Input: part model. Units: mm. Frame: model coordinates. Face numbers are marked on the shaded views. A direction names the side the tool comes from. Coordinates: 2 decimals unless noted, no trailing zeros. Write each loop counter-clockwise with the first axis right and the second up, starting at its lowest first coordinate (ties: lowest second). Pieces come first, ordered by that corner, then holes. Notation, with made-up numbers: M -2.75,24.5 L 14.25,24.5 A9 ccw 14.25,34.5 Z; hole C 26.5,47 d7. An arc over 180 degrees is marked long. Write each question's results on one line, items separated by ' | '. Start each with the question number.
1. Section query A-A, the plane x = 33. Output: boundary loops of the cut face in (y, z), and give its area (3 significant figures).
2. Ray query, probe 1 along Z at (x, y) = (15, -3); probe 2 along X at (y, z) = (-2.25, 6.25); probe 3 along Z at (x, y) = (30, 0). Return the intervals inside material, ascending.
3. Set-up query: the marked faces 1 and 2. Return all of +Z, -Z, +X, -X, +Y, -Y with unobstructed straight access to the full face (end or side cutting, diameter ignored); none if empty.
4. First-contact query: pin 1 (2 mm diameter, centred on x = 41, y = -2, fed in from -Z); pin 2 (4 mm diameter, centred on y = 3, z = -6, fed in from +X); pin 3 (5 mm diameter, centred on x = 15.5, z = 1.5, fed in from -Y). Flat tips, straight axial feed; report the tip coordinate or a pass-through.
Autodesk Inventor part; units mm, degrees
ref_plane "Work Plane1" through (1.525, 0, 0) normal (0, 0, 1) x (1, 0, 0)
ref_plane "YZ Plane" through (0, 0, 0) normal (1, 0, 0) x (0, 1, 0)
ref_plane "XZ Plane" through (0, 0, 0) normal (0, 1, 0) x (-1, 0, 0)
sketch "Sketch1" plane through (0, 0, 0) normal (0, 0, 1) x (1, 0, 0)
  line L0 (0, 7.315) -> (0, 5)
  line L1 (4.5, 5) -> (50, 5)
  line L2 (50, 5) -> (50, 0)
  line L3 (50, 0) -> (-0.6001, 0)
  line L4 (-10.7201, 0) -> (60.12, 0)
  line L5 (-0.6001, 0) -> (-0.6001, 7.315)
  line L6 (-0.6001, 7.315) -> (0, 7.315)
  line L7 (4.5, 5) -> (3.5797, 5)
  line L8 (3.5797, 5) -> (0, 5)
  line L9 (0, -1.463) -> (0, 8.778)
  dimension "d0" = 50
  dimension "d1" = 45.5
  dimension "d2" = 10
  dimension "d9" = 0.6001
  dimension "d10" = 14.63
  dimension "d13" = 0.9203
  dimension "d14" = 10
revolve "Body" add sketch "Sketch1" angle 360 about axis through (50, 0, 0) along (-1, 0, 0)
sketch "Sketch2" plane through (-0.6001, 0, 0) normal (-1, 0, 0) x (0, 0, 1)
  line L0 (0, 9.2376) -> (8, 4.6188)
  line L1 (8, 4.6188) -> (8, -4.6188)
  line L2 (8, -4.6188) -> (0, -9.2376)
  line L3 (0, -9.2376) -> (-8, -4.6188)
  line L4 (-8, -4.6188) -> (-8, 4.6188)
  line L5 (-8, 4.6188) -> (0, 9.2376)
  point P0 (0, 0)
  point P1 (0, 0)
  dimension "d11" = 16
extrude "Head" add sketch "Sketch2" along normal blind 5.8
sketch "Sketch4" plane through (0, 0, 0) normal (0, 0, 1) x (1, 0, 0)
  line L0 (-6.4001, 8) -> (-6.4001, 9.2376)
  line L1 (-6.4001, 9.2376) -> (-5.6856, 9.2376)
  line L2 (-5.6856, 9.2376) -> (-6.4001, 8)
  line L3 (-7.5601, 0) -> (0.5599, 0)
  line L4 (-0.6001, 9.2376) -> (-6.4001, 9.2376)
  line L5 (-6.4001, 4.6188) -> (-6.4001, 9.2376)
  dimension "d5" = 30
  dimension "d19" = 16
revolve "Chamfer1" cut sketch "Sketch4" angle 360 about axis through (-10, 0, 0) along (1, 0, 0)
thread "Thread"
chamfer "Chamfer2" distance 0.9202 distance2 0.9203 1 edges at (50, -5, 0) measured on face at (50, -1.8775, 0.7745)
ref_plane "Work Plane1" through (1.525, 0, 0) normal (0, 0, 1) x (1, 0, 0)
equation "\"d0\" = NLG"
equation "\"d1\" = GEL"
equation "\"d2\" = GD"
equation "\"d10\" = SD2"
equation "\"d14\" = BDM"
equation "\"d11\" = SW"
equation "\"d3\" = KOH - SD"
equation "\"d5\" = ANG1"
equation "\"d19\" = SW0"
equation "\"d15\" = GEL"
equation "\"d6\" = -0.5 * SPD + 0.5 * GD"
equation "\"NLG\" = 50"
equation "\"GD\" = NND"
equation "\"BDM\" = NND"
equation "\"KOH\" = 6.4"
equation "\"GEL\" = 45.5"
equation "\"SW\" = 16"
equation "\"SW0\" = SW"
equation "\"SPD\" = NND - 1.2269 * PTC"
equation "\"SD2\" = 14.63"
equation "\"SD\" = 0.6"
equation "\"ANG1\" = 30deg"
equation "\"GAL\" = 0.61345 * PTC"
equation "\"GUL\" = 0.61345 * PTC"
equation "\"RR\" = 0.4"
equation "\"GD1\" = THREADDIA - 1.2269 * PTC"
equation "\"SDH\" = SD2"
equation "\"SDHG\" = 4.5"
equation "\"TOA\" = 30deg"
equation "\"PTC\" = 1.5"
equation "\"E0\" = 18.48"
properties part number "ISO 4017 - M10 x 50" material "Steel, Mild"
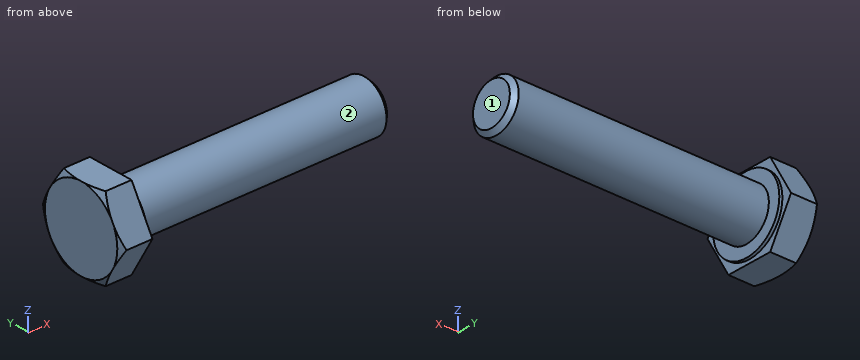
Answer:
1) outline: C 0,0 d10 | area: 78.5 mm^2
2) probe 1: -4 to 4 | probe 2: -6.4 to 0 | probe 3: -5 to 5
3) face 1: +Z, -Z, +X, +Y, -Y | face 2: +X
4) pin 1: z = -4.9 | pin 2: x = 49.37 | pin 3: y = -5
